Verification items for the finished model (mm, model axes). Round coordinates to 2 decimals unless told otherwise and drop trailing zeros. Write each loop counter-clockwise with the first axis right and the second up, starting at its lowest first coordinate (ties: lowest second). Pieces come first, ordered by that corner, then holes. Notation, with made-up numbers: M 32,39 L 67,39 A16 cw 67,70 Z; hole C 31,77.25 d2. An arc over 180 degrees is marked long. One line per question, with ' | ' between items.
from build123d import *

# Parameters (mm, degrees)
F0_W     = 76.2
F0_H     = 323.85
F1_DEPTH = 25.4
F2_DEPTH = 50.8
F0_W_2   = 50.8
F0_H_2   = 50.8
F3_DEPTH = 1574.8


with BuildPart() as f1:
    # F0 (on Top) → F1 (new body)
    with BuildSketch(Plane.XY):
        Polygon((0, 233.196965), (0, 156.996965), (736.6, 156.996965), (812.8, 156.996965), (812.8, 233.196965), align=None)
        with Locations((774.7, -4.928035)):
            Rectangle(F0_W, F0_H)
        Polygon((812.8, -166.853035), (736.6, -166.853035), (0, -166.853035), (0, -243.053035), (812.8, -243.053035), align=None)
    extrude(amount=F1_DEPTH)

    # F0 (on Top) → F2 (join)
    with BuildSketch(Plane.XY):
        Polygon((0, 20.471965), (0, 156.996965), (0, 233.196965), (-50.8, 233.196965), (-50.8, -243.053035), (0, -243.053035), (0, -166.853035), (0, -30.328035), align=None)
    extrude(amount=F2_DEPTH)

    # F0 (on Top) → F3 (join)
    with BuildSketch(Plane.XY):
        with Locations((25.4, -4.928035)):
            Rectangle(F0_W_2, F0_H_2)
    extrude(amount=F3_DEPTH)


solid = f1.part
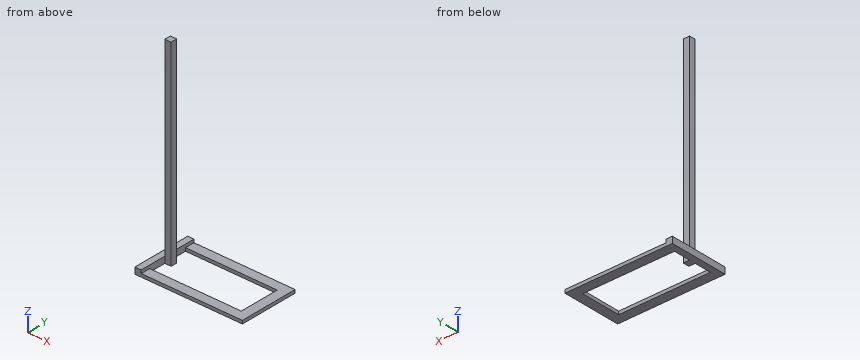
1. Thickness scan on line 1 (Z direction, x = 660, y = -184.5); line 2 (X direction, y = -30, z = 196). Record the ranges inside material, lowest first.
Results:
line 1: z = 0 to 25.4 | line 2: x = 0 to 50.8
2. Section check D-D, the plane z = 1265. Record the cut outline in (x, y).
Results:
outline: M 0,-30.33 L 50.8,-30.33 L 50.8,20.47 L 0,20.47 Z
3. Go/stop test with flat-tipped pins: P1, Ø5, axis at x = 546, y = 181.5, coming from the -Z side; P2, Ø15, axis at y = -8.5, z = 1064.5, coming from the -X side; P3, Ø15, axis at y = 1, z = 1113.5, coming from the +X side; P4, Ø15, axis at x = -15.5, y = 106, coming from the +Z side. Record where each tip stops, or that it passes through.
Results:
P1: stops at z = 0 | P2: stops at x = 0 | P3: stops at x = 50.8 | P4: stops at z = 50.8
4. Section check B-B, the plane x = 200. Record the cut outline in (y, z).
Results:
outline: M -243.05,0 L -166.85,0 L -166.85,25.4 L -243.05,25.4 Z; M 157,0 L 233.2,0 L 233.2,25.4 L 157,25.4 Z
5. Section check A-A, the plane y = -101.5. Record the cut outline in (x, z).
Results:
outline: M -50.8,0 L 0,0 L 0,50.8 L -50.8,50.8 Z; M 736.6,0 L 812.8,0 L 812.8,25.4 L 736.6,25.4 Z
6. Section check C-C, the plane y = -10. Record the cut outline in (x, z), then the cut area to 3 significant figures.
Results:
outline: M -50.8,0 L 50.8,0 L 50.8,1574.8 L 0,1574.8 L 0,50.8 L -50.8,50.8 Z; M 736.6,0 L 812.8,0 L 812.8,25.4 L 736.6,25.4 Z | area: 84,500 mm2
